CAD build for the part. Positions are in the model's coordinates, mm. A direction names the side the tool comes from. Coordinates: 2 decimals unless noted, no trailing zeros. Order: outer loops, then holes, each group sorted by start corner. A loop starts at its lowest first (then second) coordinate and runs counter-clockwise, first axis right, second up. Notation, with made-up numbers: (45.5, -32.5) - (93.5, -32.5) arc R10 cw to (93.5, -26.5) - close; hole circle Ø10 at (-9.75, -31). An arc over 180 degrees is marked (long way). Use one line per item in the form item = value.
```python
from build123d import *

# Parameters (mm, degrees)
F1_DEPTH = 127
F2_R     = 6.35
F3_DEPTH = 6.35
F4_R     = 6.35
F5_DEPTH = 6.35


with BuildPart() as f1:
    # F0 (on Right) → F1 (new body, symmetric)
    with BuildSketch(Plane.YZ):
        Polygon((38.1, 38.1), (-38.1, 38.1), (-38.1, 31.75), (31.75, 31.75), (31.75, -38.1), (38.1, -38.1), align=None)
    extrude(amount=F1_DEPTH, both=True)

    # F2 (on face) → F3 (cut, through all)
    with BuildSketch(Plane(origin=(0, 38.1, 0), x_dir=(-1, 0, 0), z_dir=(0, 1, 0))):
        with Locations((-101.6, -12.7)):
            Circle(F2_R)
        with Locations((101.6, -12.7)):
            Circle(F2_R)
    extrude(amount=-F3_DEPTH, mode=Mode.SUBTRACT)

    # F4 (on face) → F5 (cut, through all)
    with BuildSketch(Plane.XY.offset(38.1)):
        with Locations((-101.6, 3.175)):
            Circle(F4_R)
        with Locations((101.6, 3.175)):
            Circle(F4_R)
    extrude(amount=-F5_DEPTH, mode=Mode.SUBTRACT)


solid = f1.part
```
Item 1: Two-plate mould, pull along Z, no slides. Class faces 3 (the face through (107.657, 5.082, 34.969)), 4 (the face through (2, 1, 38.1)), 5 (the face through (-107.466, 34.969, -15.132)): +Z half, -Z half, draft (parallel to the pull), parting line (faces both ways), or undercut.
Derived:
face_3 = draft
face_4 = +Z half
face_5 = undercut
Item 2: Cut at C-C, the plane y = -0.5. Write the cut outline in (x, z), plus the area to 3 significant figures.
Derived:
outline = (-127, 31.75) - (-106.78, 31.75) - (-106.78, 38.1) - (-127, 38.1) - close; (-96.42, 31.75) - (96.42, 31.75) - (96.42, 38.1) - (-96.42, 38.1) - close; (106.78, 31.75) - (127, 31.75) - (127, 38.1) - (106.78, 38.1) - close
area = 1,480 mm²
Item 3: Cut at A-A, the plane x = 101.6. Write the cut outline in (y, z) (3 decimals), plus the area to 3 significant figures.
Derived:
outline = (-38.1, 31.75) - (-3.175, 31.75) - (-3.175, 38.1) - (-38.1, 38.1) - close; (9.525, 31.75) - (31.75, 31.75) - (31.75, -6.35) - (38.1, -6.35) - (38.1, 38.1) - (9.525, 38.1) - close; (31.75, -38.1) - (38.1, -38.1) - (38.1, -19.05) - (31.75, -19.05) - close
area = 766 mm²
Item 4: Drop flat-ended pins along their axis: pin 1 (5 mm diameter, centred on x = -63.5, y = -2.5, fed in from -Z); pin 2 (5 mm diameter, centred on x = -18.5, z = 0, fed in from -Y). Give the stop position or say it passes through.
Derived:
pin_1 = 31.75
pin_2 = 31.75
Item 5: Cut at D-D, the plane x = -23.5. Write the cut outline in (y, z).
Derived:
outline = (-38.1, 31.75) - (31.75, 31.75) - (31.75, -38.1) - (38.1, -38.1) - (38.1, 38.1) - (-38.1, 38.1) - close
Item 6: 3-axis set-ups, long thin cutter, end or side, ignore diameter. For faces 1 (the face through (2, -4, 31.75)), 2 (the face through (127, 17, 34)): which of +Z, -Z, +X, -X, +Y, -Y reach the whole face in a straight line?
Derived:
face_1 = -Z, +X, -X, -Y
face_2 = +Z, -Z, +X, +Y, -Y
Item 7: Cut at B-B, the plane z = -12.7. Write the cut outline in (x, y), plus the area to 3 significant figures.
Derived:
outline = (-127, 31.75) - (-107.95, 31.75) - (-107.95, 38.1) - (-127, 38.1) - close; (-95.25, 31.75) - (95.25, 31.75) - (95.25, 38.1) - (-95.25, 38.1) - close; (107.95, 31.75) - (127, 31.75) - (127, 38.1) - (107.95, 38.1) - close
area = 1,450 mm²
Item 8: Drill centre lines: line 1 (X direction, y = 35, z = -12); line 2 (Z direction, x = -101, y = 36); line 3 (X direction, y = 35, z = -18). Where is each one in solid material? Low to high. Write a range as [from, to].
Derived:
line_1 = [-127, -107.91], [-95.29, 95.29], [107.91, 127]
line_2 = [-38.1, -19.02], [-6.38, 38.1]
line_3 = [-127, -105.1], [-98.1, 98.1], [105.1, 127]
